Could you check a few things on this drawing? It's one solid part, dimensions in mm from its lowest x, y, z. Coordinates: 2 decimals unless noted, no trailing zeros. Loops run counter-clockwise (first coordinate to the right, second up) from the corner with the lowest first, then second, coordinate; pieces in that order, holes last.
1) Thinking about a two-plate mould opening in X: for the marked faces 1, 2, 3 and 4, which applies, released by +X, released by -X, zero draft, split by the parting line, or undercut?
2) Imagine slicing it at B-B on y = 121. Please give me the cut outline in (x, z), plus the area to 3 significant figures.
3) Imagine slicing it at C-C on x = 50. Please give me the cut outline in (y, z).
4) If I drill on line 1 along Y through (x, z) = (118, 9.5); line 2 along X through (y, z) = (98.5, 37); line 3 along X through (y, z) = (147, 38.5), over which ranges is the centre line in solid material (lowest first)?
5) Imagine slicing it at A-A on z = 40. Please give me the cut outline in (x, y), plus the area to 3 significant figures.
6) Imagine slicing it at D-D on z = 118.5. Please give me the cut outline in (x, y), plus the area to 3 significant figures.
7) Will this pin go through, and if not, where does the flat tip stop? P1, Ø12, axis at x = 77, z = 45, coming from the +Y side.
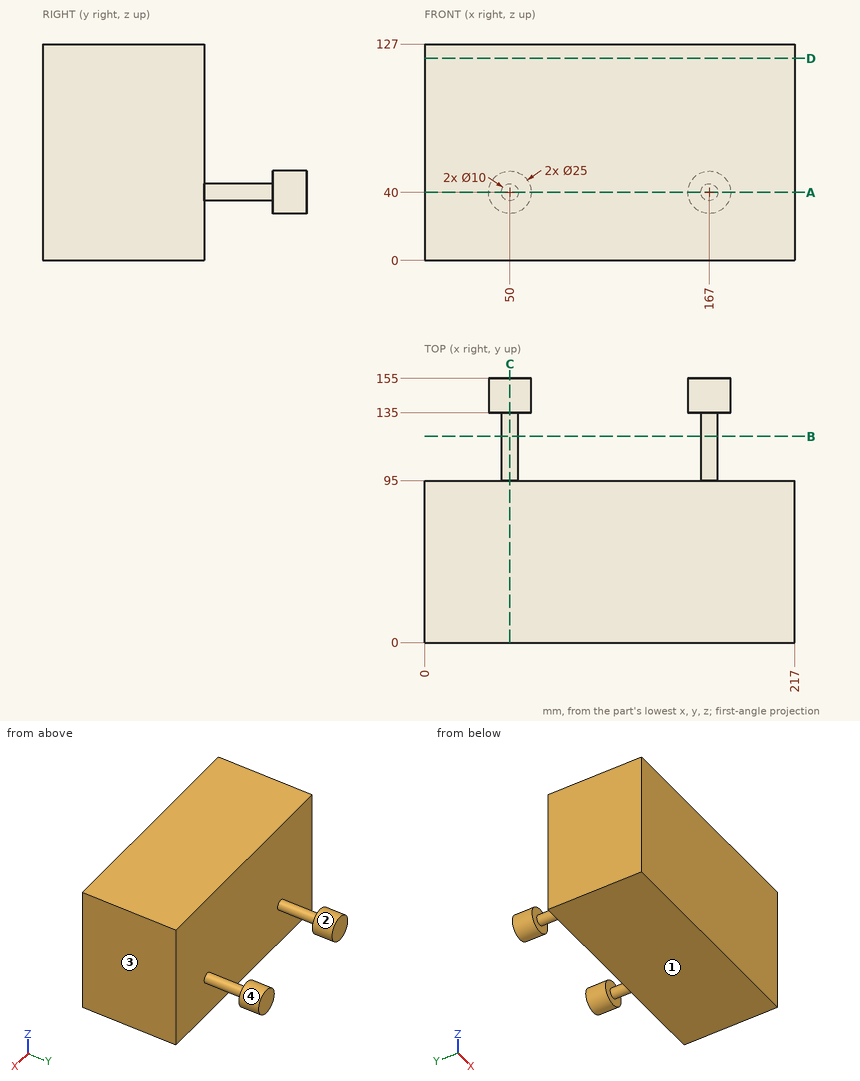
Filled in:
1. face 1: zero draft
1. face 2: undercut
1. face 3: released by +X
1. face 4: undercut
2. outline: circle Ø10 at (50, 40); circle Ø10 at (167, 40)
2. area: 157 mm2
3. outline: (0, 0) - (95, 0) - (95, 35) - (135, 35) - (135, 27.5) - (155, 27.5) - (155, 52.5) - (135, 52.5) - (135, 45) - (95, 45) - (95, 127) - (0, 127) - close
4. line 1: y = 0 to 95
4. line 2: x = 46 to 54, 163 to 171
4. line 3: x = 37.59 to 62.41, 154.59 to 179.41
5. outline: (0, 0) - (217, 0) - (217, 95) - (172, 95) - (172, 135) - (179.5, 135) - (179.5, 155) - (154.5, 155) - (154.5, 135) - (162, 135) - (162, 95) - (55, 95) - (55, 135) - (62.5, 135) - (62.5, 155) - (37.5, 155) - (37.5, 135) - (45, 135) - (45, 95) - (0, 95) - close
5. area: 22,400 mm2
6. outline: (0, 0) - (217, 0) - (217, 95) - (0, 95) - close
6. area: 20,600 mm2
7. P1: stops at y = 95
